For this review, take the finished solid that the model builds, in its own axes (mm). Face numbers are marked on the shaded views. A direction names the side the tool comes from. Round coordinates to 2 decimals unless told otherwise and drop trailing zeros. Order: outer loops, then holes, each group sorted by start corner. A loop starts at its lowest first (then second) coordinate and runs counter-clockwise, first axis right, second up. Notation, with made-up numbers: M 26.5,61 L 49.5,61 A9 cw 49.5,70 Z; hole C -35.75,-34 d10. An arc over 180 degrees is marked long. Answer as a JSON object with one key per item and string values.
from build123d import *

# Parameters (mm, degrees)
SKETCH1_W           = 120
SKETCH1_H           = 80
BOSS_EXTRUDE1_DEPTH = 90
CUT_EXTRUDE1_DEPTH  = 90
CUT_EXTRUDE2_DEPTH  = 90
CUT_EXTRUDE3_DEPTH  = 90
CUT_EXTRUDE4_DEPTH  = 90
CUT_EXTRUDE5_DEPTH  = 90


with BuildPart() as part:
    # Sketch1 → Boss-Extrude1 (new body)
    with BuildSketch(Plane.XY):
        with Locations((60, 40)):
            Rectangle(SKETCH1_W, SKETCH1_H)
    extrude(amount=-BOSS_EXTRUDE1_DEPTH)

    # Sketch2 → Cut-Extrude1 (cut)
    with BuildSketch(Plane.XY):
        Polygon((0, 40), (10, 40), (40, 70), (100, 70), (100, 80), (0, 80), align=None)
    extrude(amount=-CUT_EXTRUDE1_DEPTH, mode=Mode.SUBTRACT)

    # Sketch3 → Cut-Extrude2 (cut)
    with BuildSketch(Plane.XZ):
        Polygon((0, -60), (10, -60), (30, -50), (30, -20), (90, -20), (110, 0), (0, 0), align=None)
    extrude(amount=-CUT_EXTRUDE2_DEPTH, mode=Mode.SUBTRACT)

    # Sketch4 → Cut-Extrude3 (cut)
    with BuildSketch(Plane(origin=(0, 20, 0), x_dir=(1, 0, 0), z_dir=(0, 1, 0))):
        Polygon((30, 20), (30, 50), (50, 40), (70, 40), (90, 20), align=None)
    extrude(amount=CUT_EXTRUDE3_DEPTH, mode=Mode.SUBTRACT)

    # Sketch5 → Cut-Extrude4 (cut)
    with BuildSketch(Plane(origin=(0, 40, 0), x_dir=(1, 0, 0), z_dir=(0, 1, 0))):
        Polygon((70, 40), (70, 70), (10, 70), (10, 60), (50, 40), align=None)
    extrude(amount=CUT_EXTRUDE4_DEPTH, mode=Mode.SUBTRACT)

    # Sketch6 → Cut-Extrude5 (cut)
    with BuildSketch(Plane.XY.offset(-70)):
        Polygon((70, 40), (100, 70), (70, 70), align=None)
    extrude(amount=CUT_EXTRUDE5_DEPTH, mode=Mode.SUBTRACT)


solid = part.part
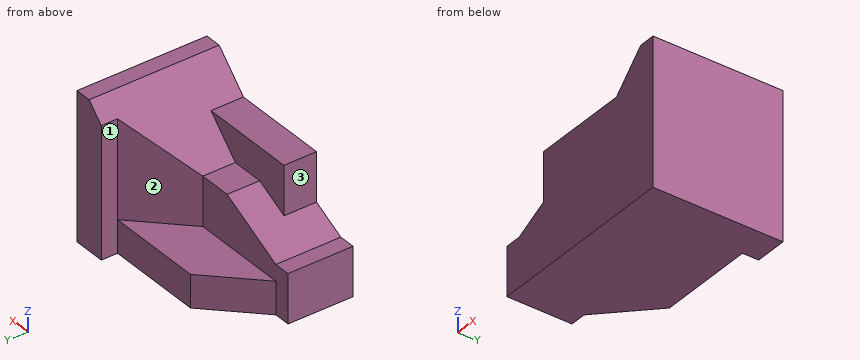
1) Machinability: for the marked faces 1, 2 and 3, which of the approach directions +Z, -Z, +X, -X, +Y, -Y give a long, thin tool a straight path to every point of the face, cutting with its end or side? Answer none if there is none.
Geometry check:
{"face 1": "+Z, -Z, -X, +Y", "face 2": "+Z, -X, +Y", "face 3": "+Z, -X, +Y, -Y"}
2) Insertion check: P1, Ø5, axis at y = 61.5, z = -26, coming from the -X side; P2, Ø8, axis at x = 7, y = 14.5, coming from the +Z side; P3, Ø1, axis at x = 100.5, y = 54.5, coming from the +Z side. Each pin has a flat end and moves straight along its axis. Give the tip position at first contact, or say it passes through.
Geometry check:
{"P1": "stops at x = 89", "P2": "stops at z = -59.5", "P3": "stops at z = -9"}
3) Add section C-C on x = 21. State the section outline as (y, z) points.
Geometry check:
{"outline": "M 0,-90 L 51,-90 L 51,-70 L 40,-70 L 40,-54.5 L 0,-54.5 Z"}
4) For L1, parallel to Z at x = 22.5, y = 52; L2, parallel to Z at x = 52.5, y = 36; L3, parallel to Y at x = 62.5, z = -59.5, list the stretches that pass through material, from the lowest coordinate up.
Geometry check:
{"L1": "z = -90 to -70", "L2": "z = -90 to -40", "L3": "y = 0 to 40"}
5) Add section D-D on z = -84. State the section outline as (x, y) points, and give its area (3 significant figures).
Geometry check:
{"outline": "M 0,0 L 120,0 L 120,80 L 100,80 L 100,70 L 40,70 L 10,40 L 0,40 Z", "area": "7,850 mm²"}
6) Add section A-A on z = -28.5. State the section outline as (x, y) points, and give its area (3 significant figures).
Geometry check:
{"outline": "M 30,0 L 120,0 L 120,80 L 100,80 L 100,70 L 81.5,51.5 L 81.5,20 L 30,20 Z", "area": "3,750 mm²"}
7) Add section B-B on y = 59.5. State the section outline as (x, z) points, and give its area (3 significant figures).
Geometry check:
{"outline": "M 29.5,-90 L 120,-90 L 120,0 L 110,0 L 89.5,-20.5 L 89.5,-70 L 29.5,-70 Z", "area": "3,730 mm²"}
